Design review of the part built by this model. Coordinates are the model's own, in mm. A direction names the side the tool comes from. Give positions to 0.01 mm unless a question says otherwise; leave off trailing zeros. Loops run counter-clockwise (first coordinate to the right, second up) from the corner with the lowest first, then second, coordinate; pieces in that order, holes last. Notation, with made-up numbers: M -4,-2.75 L 36,-2.75 A21 cw 36,28.25 Z; hole C 9.25,21.25 d8. An arc over 180 degrees is marked long. Answer as CSV lines item,"result".
Autodesk Inventor part; units mm, degrees
ref_plane "YZ Plane" through (0, 0, 0) normal (1, 0, 0) x (0, 1, 0)
ref_plane "XZ Plane" through (0, 0, 0) normal (0, 1, 0) x (-1, 0, 0)
ref_plane "XY Plane" through (0, 0, 0) normal (0, 0, 1) x (1, 0, 0)
sketch "Sketch2" plane through (0, 0, 0) normal (0, 1, 0) x (-1, 0, 0)
  line L0 (0, 0) -> (0, -65)
  line L1 (0, 0) -> (22, 0)
  line L2 (22, 0) -> (22, -40.3)
  line L3 (22, -40.3) -> (0, -65)
  dimension "d4" = 65
  dimension "d5" = 22
  dimension "d6" = 40.3
revolve "Revolution1" add sketch "Sketch2" angle 360 about axis through (0, 0, 0) along (-1, 0, 0)
sketch "Sketch3" plane through (-22, 0, 0) normal (-1, 0, 0) x (0, 0, 1)
  circle A0 centre (0, 0) radius 40.3
  line L0 (0, 40.3) -> (0, 64.3)
  line L1 (0, 64.3) -> (-7.5, 64.3)
  line L2 (-7.5, 64.3) -> (-7.5, 45.231)
  line L3 (0, 64.3) -> (7.4, 64.3)
  line L4 (7.4, 64.3) -> (7.4771, 45.2525)
  arc A1 (2.2037, 40.2397) -> (-2.2241, 40.2386) centre (0, 0) ccw
  arc A2 (-7.5, 45.231) -> (-2.2241, 40.2386) centre (-2.5, 45.231) ccw
  arc A3 (2.2037, 40.2397) -> (7.4771, 45.2525) centre (2.4771, 45.2322) ccw
  point P0 (-7.5, 39.596)
  point P1 (7.5, 39.596)
  dimension "d11" = 24
  dimension "d12" = 7.5
  dimension "d13" = 7.4
  dimension "d17" = 5
extrude "Extrusion1" cut sketch "Sketch3" against normal blind 10 contours A0 L0 L3 L4 A3 | A2 L2 L1 L0 A0
sketch "Sketch4" plane through (-22, 0, 0) normal (-1, 0, 0) x (0, 0.0003, 1)
  point P0 (0, 0)
sketch "Sketch6" plane through (-12, 0, 0) normal (-1, 0, 0) x (0, 0, 1)
  point P0 (0, 0)
sketch "Sketch7" plane through (-22, 0, 0) normal (-1, 0, 0) x (0, 0.0003, 1)
  point P0 (0, 0)
sketch "Sketch8" plane through (0, 0, 0) normal (1, 0, 0) x (0, 0, -1)
  circle A0 centre (0, 0) radius 65
extrude "Extrusion2" add sketch "Sketch8" along normal blind 3
sketch "Sketch10" plane through (-22, 0, 0) normal (-1, 0, 0) x (0, 0.0003, 1)
  line L0 (0, 0) -> (-112.4723, 0)
  line L1 (-112.4723, 0) -> (-112.4723, -208.2132)
  line L2 (-112.4723, -208.2132) -> (0, -208.2132)
  line L3 (0, -208.2132) -> (0, 0)
properties part number "Handle Gearbox" material "PC/ABS Plastic"
1. For faces 1 (the flat face through (-22, -1, 1)), 2 (the cylindrical face through (-17.1, 40.3, 0)), list the 3-axis set-ups (+Z, -Z, +X, -X, +Y, -Y) from which the entire face can be reached by the end or side of a thin tool; tool diameter is ignored.
Answer block:
face 1,"+Z, -Z, -X, +Y, -Y"
face 2,"-X, +Y"
2. We need section A-A, the plane z = 0. Write out the cut boundary in (x, y), plus the area to 3 significant figures.
Answer block:
outline,"M -22,-40.3 L 0,-65 L 3,-65 L 3,65 L 0,65 L -12,51.53 L -12,40.3 L -22,40.3 Z"
area,"2,650 mm²"
3. We need section C-C, the plane x = -19.75. Write out the cut boundary in (y, z).
Answer block:
outline,"M 40.24,-2.22 A40.3 ccw 40.24,2.2 A5 cw 42.32,6.54 A42.83 ccw long 42.32,-6.57 A5 cw Z"
4. For P1, Ø3, axis at x = -8, z = 17.5, coming from the -Y side; P2, Ø2, axis at x = -3.5, z = -50.5, coming from the +Y side; P3, Ø5.5, axis at y = 45, z = 1, coming from the -X side, all flat-tipped, find the tip position at first contact; note any pin that passes through.
Answer block:
P1,"y = -55.05"
P2,"y = 36.74"
P3,"x = -12"
5. We need section D-D, the plane x = -10. Write out the cut boundary in (y, z), plus the area to 3 significant figures.
Answer block:
outline,"C 0,0 d107.55"
area,"9,080 mm²"
6. We need section B-B, the plane y = 0. Write out the cut boundary in (x, z), plus the area to 3 significant figures.
Answer block:
outline,"M -22,-40.3 L 0,-65 L 3,-65 L 3,65 L 0,65 L -22,40.3 Z"
area,"2,710 mm²"
7. To check wall thickness, follow L1, parallel to Z at x = -7, y = -18; L2, parallel to Y at x = 1.25, z = -11; L3, parallel to X at y = -45, z = 28. State the ranges of each line that lie inside material, in increasing order. Write a range as [from, to].
Answer block:
L1,"[-54.23, 54.23]"
L2,"[-64.06, 64.06]"
L3,"[-10.69, 3]"
8. The part is to be moulded in two halves that separate along Z. For faces 3 (the flat face through (-12, 46, 0)), 4 (the flat face through (3, 1, 1)), 5 (the conical face through (-20.624, -40.85, 9.071)), say which applies: pulls with the +Z half, pulls with the -Z half, needs draft (parallel to the pull), parting line crosses it, or undercut.
Answer block:
face 3,"undercut"
face 4,"needs draft"
face 5,"parting line crosses it"
